```python
from build123d import *

# Parameters (mm, degrees)
SKETCH1_W           = 228.6
SKETCH1_H           = 38.1
BOSS_EXTRUDE1_DEPTH = 12.7
SHELL1_T            = -3.175
SKETCH3_W           = 3.175
SKETCH3_H           = 31.75
CUT_EXTRUDE1_DEPTH  = 9.525
SKETCH4_W           = 25.4
SKETCH4_H           = 16.383
SKETCH4_W_2         = 31.75
SKETCH4_H_2         = 17.526
SKETCH4_W_3         = 38.1
SKETCH4_H_3         = 19.685
SKETCH4_W_4         = 44.45
SKETCH4_H_4         = 22.733
CUT_EXTRUDE2_DEPTH  = 232.948907359


with BuildPart() as part:
    # Sketch1 → Boss-Extrude1 (new body)
    with BuildSketch(Plane(origin=(0, 0, 0), x_dir=(1, 0, 0), z_dir=(0, 1, 0))):
        with Locations((114.3, 19.05)):
            Rectangle(SKETCH1_W, SKETCH1_H)
    extrude(amount=-BOSS_EXTRUDE1_DEPTH)

    # Shell1
    shell1_openings = [part.faces().sort_by_distance(p)[0] for p in [
        (114.3, 0, -19.05),
    ]]
    offset(amount=SHELL1_T, openings=shell1_openings, kind=Kind.INTERSECTION)

    # Sketch3 → Cut-Extrude1 (cut)
    with BuildSketch(Plane(origin=(0, 0, 0), x_dir=(1, 0, 0), z_dir=(0, 1, 0))):
        with Locations((227.0125, 19.05)):
            Rectangle(SKETCH3_W, SKETCH3_H)
    extrude(amount=-CUT_EXTRUDE1_DEPTH, mode=Mode.SUBTRACT)

    # Sketch4 → Cut-Extrude2 (cut, through all)
    with BuildSketch(Plane(origin=(0, -9.525, 0), x_dir=(1, 0, 0), z_dir=(0, 1, 0))):
        with Locations((209.55, 13.2715)):
            Rectangle(SKETCH4_W, SKETCH4_H)
        with Locations((155.575, 13.843)):
            Rectangle(SKETCH4_W_2, SKETCH4_H_2)
        with Locations((95.25, 14.9225)):
            Rectangle(SKETCH4_W_3, SKETCH4_H_3)
        with Locations((28.575, 16.4465)):
            Rectangle(SKETCH4_W_4, SKETCH4_H_4)
    extrude(amount=-CUT_EXTRUDE2_DEPTH, mode=Mode.SUBTRACT)


solid = part.part
```
Here's how the part is built. I have some questions about the finished solid (model axes, mm). A direction names the side the tool comes from. Round coordinates to 2 decimals unless told otherwise and drop trailing zeros. Loops run counter-clockwise (first coordinate to the right, second up) from the corner with the lowest first, then second, coordinate; pieces in that order, holes last. Notation, with made-up numbers: (46.25, 34.5) -> (78.25, 34.5) arc R28 ccw to (78.25, 53.5) -> close; hole circle Ø9 at (3, 59.25). An arc over 180 degrees is marked (long way). Answer as CSV lines item,"result". Start each with the question number.
1. I'm going to push flat-ended pins straight in: P1, Ø6, axis at x = 113, z = -27.5, coming from the +Y side (3 decimals); P2, Ø3, axis at x = 108, y = -4.5, coming from the +Z side; P3, Ø3, axis at y = -3.5, z = -13.5, coming from the +X side (3 decimals); P4, Ø4, axis at x = 111.5, z = -20, coming from the +Y side. Where does each tip first touch, or does it pass through?
2. Imagine slicing it at C-C on x = 129.5. Write out the boundary of the cut face in (y, z) (3 decimals).
3. If we mould it in two halves opening along Z, with no side actions, what happens to faces 1 (the face through (3.175, -5, -19)), 2 (the face through (113, -6, 0)), 3 (the face through (113, -6, -38.1))? For each: pulls with the +Z half, pulls with the -Z half, needs draft (parallel to the pull), parting line crosses it, or undercut.
4. Imagine slicing it at D-D on y = -3.5. Write out the boundary of the cut face in (x, z) (3 decimals), plus the area to 3 significant figures.
5. Imagine slicing it at A-A on z = -11.5. Write out the boundary of the cut face in (x, y) (3 decimals).
6. I need wall thicknesses on probe 1 along X at (y, z) = (-10.25, -24.5); probe 2 along X at (y, z) = (-11.25, -18); probe 3 along Z at (x, y) = (35, -5.5) (3 decimals). Which ranges of each line are inside material? Lowest first, please. Write a range as from..to.
7. For faces 4 (the face through (139, -9.525, -23)), 5 (the face through (228.6, -10, -19)), which set-ups out of +Z, -Z, +X, -X, +Y, -Y let a thin tool reach every point of the face, with its end or its side?
8. Imagine slicing it at B-B on x = 34. Write out the boundary of the cut face in (y, z) (3 decimals), plus the area to 3 significant figures.
Solution:
1,P1,"y = -9.525"
1,P2,"z = 0"
1,P3,"x = 3.175"
1,P4,"through"
2,outline,"(-12.7, -38.1) -> (0, -38.1) -> (0, -34.925) -> (-9.525, -34.925) -> (-9.525, -3.175) -> (0, -3.175) -> (0, 0) -> (-12.7, 0) -> close"
3,face 1,"undercut"
3,face 2,"pulls with the +Z half"
3,face 3,"pulls with the -Z half"
4,outline,"(0, -38.1) -> (228.6, -38.1) -> (228.6, -34.925) -> (3.175, -34.925) -> (3.175, -3.175) -> (228.6, -3.175) -> (228.6, 0) -> (0, 0) -> close"
4,area,"1,550 mm²"
5,outline,"(0, -12.7) -> (6.35, -12.7) -> (6.35, -9.525) -> (3.175, -9.525) -> (3.175, 0) -> (0, 0) -> close; (50.8, -12.7) -> (76.2, -12.7) -> (76.2, -9.525) -> (50.8, -9.525) -> close; (114.3, -12.7) -> (139.7, -12.7) -> (139.7, -9.525) -> (114.3, -9.525) -> close; (171.45, -12.7) -> (196.85, -12.7) -> (196.85, -9.525) -> (171.45, -9.525) -> close; (222.25, -12.7) -> (228.6, -12.7) -> (228.6, -9.525) -> (222.25, -9.525) -> close"
6,probe 1,"0..6.35, 50.8..76.2, 114.3..228.6"
6,probe 2,"0..6.35, 50.8..76.2, 114.3..139.7, 171.45..196.85, 222.25..228.6"
6,probe 3,"-38.1..-34.925, -3.175..0"
7,face 4,"+X, +Y"
7,face 5,"+Z, -Z, +X, +Y, -Y"
8,outline,"(-12.7, -38.1) -> (0, -38.1) -> (0, -34.925) -> (-9.525, -34.925) -> (-9.525, -27.813) -> (-12.7, -27.813) -> close; (-12.7, -5.08) -> (-9.525, -5.08) -> (-9.525, -3.175) -> (0, -3.175) -> (0, 0) -> (-12.7, 0) -> close"
8,area,"109 mm²"
